Input: part model. Units: mm. Frame: model coordinates. A direction names the side the tool comes from. Round coordinates to 2 decimals unless told otherwise and drop trailing zeros. Loops run counter-clockwise (first coordinate to the right, second up) from the corner with the lowest first, then second, coordinate; pieces in that order, holes last. Notation, with made-up numbers: (-6.75, -35) -> (20.25, -35) arc R19 ccw to (20.25, -14) -> close; hole circle Ø2 at (44.5, 42.25). An arc over 180 degrees is marked (long way). Answer as a JSON object with one key per item and string values.
```python
from build123d import *

# Parameters (mm, degrees)
SKETCH1_R          = 28.575
CONE_EXTRUDE_DEPTH = 25.4
CONE_EXTRUDE_TAPER = 25
CHAMFER1_SIZE      = 2
CHAMFER1_SIZE_2    = 4.134883836
NUT_HOLE_CUT_DEPTH = 5.08
SKETCH4_R          = 5.08
CUT_EXTRUDE2_DEPTH = 46.232329699
FILLET2_R          = 0.635


with BuildPart() as part:
    # Sketch1 → Cone Extrude (new body)
    with BuildSketch(Plane.XY):
        Circle(SKETCH1_R)
    extrude(amount=CONE_EXTRUDE_DEPTH, taper=CONE_EXTRUDE_TAPER)

    # Chamfer1
    # the kernel refuses this chamfer: 4.134883836, 2 mm, written as the material it takes off along each edge
    with BuildSketch(Plane(origin=(0, 0, 25.4), x_dir=(1, 0, 0), z_dir=(0, 1, 0))) as chamfer1_piece_1:
        Polygon((16.730785483 + CHAMFER1_SIZE * 0.422618261741, CHAMFER1_SIZE * 0.906307787037), (16.730785483 - CHAMFER1_SIZE_2, 0), (16.730785483, 0), align=None)
    revolve(axis=Axis((0, 0, 25.4), (0, 0, -1)), mode=Mode.SUBTRACT)

    # Sketch3 → Nut Hole Cut (cut)
    with BuildSketch(Plane.XY.offset(25.4)):
        Polygon((6.741570116, 5.654240212), (-1.525930605, 8.665491088), (-8.267500721, 3.011250876), (-6.741570116, -5.654240212), (1.525930605, -8.665491088), (8.267500721, -3.011250876), align=None)
    extrude(amount=-NUT_HOLE_CUT_DEPTH, mode=Mode.SUBTRACT)

    # Sketch4 → Cut-Extrude2 (cut, through all)
    with BuildSketch(Plane.XY.offset(20.32)):
        Circle(SKETCH4_R)
    extrude(amount=-CUT_EXTRUDE2_DEPTH, mode=Mode.SUBTRACT)

    # Fillet2
    fillet2_edges = [part.edges().sort_by_distance(p)[0] for p in [
        (-28.575, 0, 0),
    ]]
    fillet(fillet2_edges, radius=FILLET2_R)


solid = part.part
```
1) Reachability of faces 1 (the face through (-2.666, -7.139, 22.896)), 2 (the face through (-0.661, 5.037, 10.302)) from +Z, -Z, +X, -X, +Y, -Y: full face, straight path, thin tool, end or side. Return the list, or none.
Output:
{"face 1": "+Z", "face 2": "+Z, -Z"}
2) Draft query along Y for faces 3 (the face through (2.666, 7.139, 22.896)), 4 (the face through (-0.2, -8.2, 25.4)), 5 (the face through (-2.783, 12.532, 25.312)), 6 (the face through (4.85, -5.88, 22.9)). Return one class per face: +Y half, -Y half, draft (parallel to the pull), parting line (faces both ways), or undercut.
Output:
{"face 3": "undercut", "face 4": "draft", "face 5": "parting line", "face 6": "undercut"}
3) Section C-C, the plane z = 12. Output: boundary loops of the cut face in (x, y), plus the area to 3 significant figures.
Output:
{"outline": "circle Ø45.96 at (0, 0); hole circle Ø10.16 at (0, 0)", "area": "1,580 mm^2"}
4) Contact query for flat-ended pins moving along their axis: P1, Ø5, axis at x = 17.5, z = 21.5, coming from the +Y side; P2, Ø8, axis at y = 7.5, z = 19.5, coming from the +X side; P3, Ø5, axis at x = 1.5, y = 0, coming from the +Z side; P4, Ø4, axis at x = 11.5, y = 11.5, coming from the +Z side. Output: stop coordinate, or through.
Output:
{"P1": "stops at y = 11.44", "P2": "stops at x = 20.37", "P3": "passes through", "P4": "stops at z = 24.79"}
5) Ray query, probe 1 along Y at (x, z) = (0, 11.5); probe 2 along Y at (x, z) = (1.5, 17.75); probe 3 along Z at (x, y) = (15, -23.5). Return the intervals inside material, ascending.
Output:
{"probe 1": "y = -23.21 to -5.08, 5.08 to 23.21", "probe 2": "y = -20.24 to -4.85, 4.85 to 20.24", "probe 3": "z = 0.08 to 1.49"}
6) Section A-A, the plane x = 0. Output: boundary loops of the cut face in (y, z) (3 decimals).
Output:
{"outline": "(-28.154, 0.903) arc R0.635 ccw to (-27.578, 0) -> (-5.08, 0) -> (-5.08, 20.32) -> (-8.11, 20.32) -> (-8.11, 25.4) -> (-12.596, 25.4) -> (-17.576, 23.587) -> close; (5.08, 0) -> (27.578, 0) arc R0.635 ccw to (28.154, 0.903) -> (17.576, 23.587) -> (12.596, 25.4) -> (8.11, 25.4) -> (8.11, 20.32) -> (5.08, 20.32) -> close"}
7) Section D-D, the plane z = 2. Output: boundary loops of the cut face in (x, y).
Output:
{"outline": "circle Ø55.28 at (0, 0); hole circle Ø10.16 at (0, 0)"}
8) Section B-B, the plane y = 0. Output: boundary loops of the cut face in (x, z) (3 decimals).
Output:
{"outline": "(-28.154, 0.903) arc R0.635 ccw to (-27.578, 0) -> (-5.08, 0) -> (-5.08, 20.32) -> (-7.737, 20.32) -> (-7.737, 25.4) -> (-12.596, 25.4) -> (-17.576, 23.587) -> close; (5.08, 0) -> (27.578, 0) arc R0.635 ccw to (28.154, 0.903) -> (17.576, 23.587) -> (12.596, 25.4) -> (7.737, 25.4) -> (7.737, 20.32) -> (5.08, 20.32) -> close"}
